```python
from build123d import *

# Parameters (mm, degrees)
SKETCH_W               = 110
SKETCH_H               = 142.126704
PAD_DEPTH              = 2
SKETCH001_W            = 70
SKETCH001_H            = 60
PAD001_DEPTH           = 3
PAD002_DEPTH           = 2
LINEARPATTERN_COUNT    = 22
LINEARPATTERN_PITCH    = 6.409401
PAD003_DEPTH           = 2
LINEARPATTERN001_COUNT = 22
LINEARPATTERN001_PITCH = 6.409401


with BuildPart() as part:
    # Sketch → Pad (new body)
    with BuildSketch(Plane.XY):
        with Locations((55, -71.063352)):
            Rectangle(SKETCH_W, SKETCH_H)
    extrude(amount=PAD_DEPTH)

    # Sketch001 (on Face6 of Pad) → Pad001 (join)
    with BuildSketch(Plane.XY.offset(2)):
        with Locations((55, -84.580159)):
            Rectangle(SKETCH001_W, SKETCH001_H)
    extrude(amount=PAD001_DEPTH)

    # Sketch002 (on Face3 of Pad001) → Pad002 (join)
    with BuildSketch(Plane.YZ.offset(110)):
        Polygon((-6.309401, 0), (-5.154701, 2), (-3.154701, 2), (-2, 0), align=None)
    pad002 = extrude(amount=PAD002_DEPTH)

    # LinearPattern: Pad002 ×22
    with Locations(*[(0, -i * LINEARPATTERN_PITCH, 0) for i in range(1, LINEARPATTERN_COUNT)]):
        add(pad002)

    # Sketch003 (on Face2 of LinearPattern) → Pad003 (join)
    with BuildSketch(Plane(origin=(0, 0, 0), x_dir=(0, -1, 0), z_dir=(-1, 0, 0))):
        Polygon((2, 0), (3.154701, 2), (5.154701, 2), (6.309401, 0), align=None)
    pad003 = extrude(amount=PAD003_DEPTH)

    # LinearPattern001: Pad003 ×22
    with Locations(*[(0, -i * LINEARPATTERN001_PITCH, 0) for i in range(1, LINEARPATTERN001_COUNT)]):
        add(pad003)


solid = part.part
```
Here's how the part is built. I have some questions about the finished solid (model axes, mm). A direction names the side the tool comes from. Round coordinates to 2 decimals unless told otherwise and drop trailing zeros. Write each loop counter-clockwise with the first axis right and the second up, starting at its lowest first coordinate (ties: lowest second). Pieces come first, ordered by that corner, then holes. Notation, with made-up numbers: M 6,61 L 24,61 A37 ccw 24,98 Z; hole C 41,-1.75 d10. An arc over 180 degrees is marked long. Answer as CSV lines item,"result". Start each with the question number.
1. Suppose I cut it at B-B on z = 4.1. Write out the boundary of the cut face in (x, y), then the cut area to 3 significant figures.
2. Suppose I cut it at C-C on x = 8. Write out the boundary of the cut face in (y, z).
3. I'm going to push flat-ended pins straight in: pin 1 Ø1.5 at (x, z) = (35, 2.5) entering from +Y; pin 2 Ø0.6 at (y, z) = (-1.5, 1) entering from -X; pin 3 Ø1.6 at (y, z) = (-123, 1) entering from +X. Where does each tip first touch, or does it pass through?
4. I need wall thicknesses on probe 1 along Z at (x, y) = (70, -136); probe 2 along X at (y, z) = (-14, 1.35); probe 3 along Y at (x, z) = (78.5, 3.3). Which ranges of each line are inside material? Lowest first, please.
5. On a 3-axis mill with a long thin cutter (end or side, diameter ignored), from which of +Z, -Z, +X, -X, +Y, -Y can I reach the whole of each face in a straight line? I mean faces 1 (the flat face through (55, -84, 5)), 2 (the flat face through (90, -85, 3)), 3 (the flat face through (55, -54.58, 3)), 4 (the flat face through (20, -85, 3)), 5 (the flat face through (55, -114.58, 3)). Say none if no direction works.
6. Suppose I cut it at A-A on x = 36.5. Write out the boundary of the cut face in (y, z), then the cut area to 3 significant figures.
Check result:
1,outline,"M 20,-114.58 L 90,-114.58 L 90,-54.58 L 20,-54.58 Z"
1,area,"4,200 mm2"
2,outline,"M -142.13,0 L 0,0 L 0,2 L -142.13,2 Z"
3,pin 1,"stops at y = 0"
3,pin 2,"stops at x = 0"
3,pin 3,"stops at x = 110"
4,probe 1,"z = 0 to 2"
4,probe 2,"x = 0 to 110"
4,probe 3,"y = -114.58 to -54.58"
5,face 1,"+Z, +X, -X, +Y, -Y"
5,face 2,"+Z, +X, +Y, -Y"
5,face 3,"+Z, +X, -X, +Y"
5,face 4,"+Z, -X, +Y, -Y"
5,face 5,"+Z, +X, -X, -Y"
6,outline,"M -142.13,0 L 0,0 L 0,2 L -54.58,2 L -54.58,5 L -114.58,5 L -114.58,2 L -142.13,2 Z"
6,area,"464 mm2"
